The drawing under review shows one solid part. Ordinate dimensions are in mm from its lowest x, y, z. Round coordinates to 2 decimals unless told otherwise and drop trailing zeros. Order: outer loops, then holes, each group sorted by start corner. A loop starts at its lowest first (then second) coordinate and runs counter-clockwise, first axis right, second up. Notation, with made-up numbers: (66.5, 6.25) -> (89.5, 6.25) arc R25 cw to (89.5, 31.25) -> close; hole circle Ø11 at (-30.75, 67). An arc over 180 degrees is marked (long way). Use a Markdown table: item, result. Add a question column.
1) Consider section A-A (z = 2.5). State the section outline as (x, y) points, plus the area to 3 significant figures.
2) Wall thickness on line 1 along X through (y, z) = (3.3, 3.3); line 2 along Z through (x, y) = (18.5, 0.8); line 3 along Y through (x, z) = (15.5, 3.15): over which ranges is each line inside the solid? List them lowest first. Write a range as [from, to].
3) Consider section B-B (y = 3). State the section outline as (x, z) points.
4) Clearance check with a flat-ended pin moving along its axis: P1, Ø1.5, axis at x = 3.5, z = 3, coming from the +Y side. State where the tip first meets the part, or that it passes through.
5) Consider section C-C (x = 3.25). State the section outline as (y, z) points, plus the area to 3 significant figures.
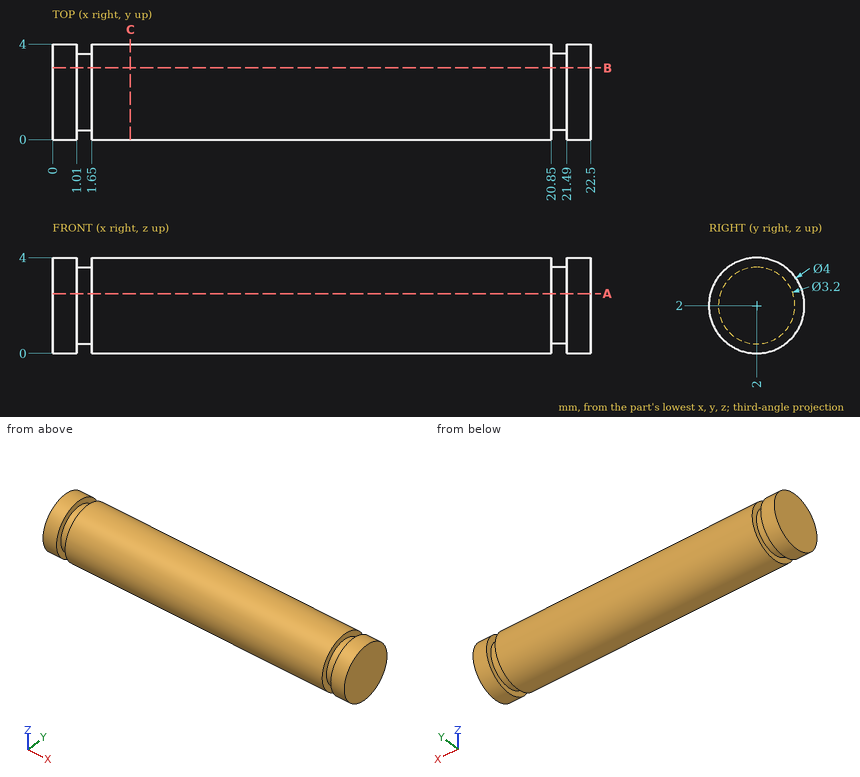
Results list:
| question | item | result |
|---|---|---|
| 1 | outline | (0, 0.06) -> (1.01, 0.06) -> (1.01, 0.48) -> (1.65, 0.48) -> (1.65, 0.06) -> (20.85, 0.06) -> (20.85, 0.48) -> (21.49, 0.48) -> (21.49, 0.06) -> (22.5, 0.06) -> (22.5, 3.94) -> (21.49, 3.94) -> (21.49, 3.52) -> (20.85, 3.52) -> (20.85, 3.94) -> (1.65, 3.94) -> (1.65, 3.52) -> (1.01, 3.52) -> (1.01, 3.94) -> (0, 3.94) -> close |
| 1 | area | 86.1 mm2 |
| 2 | line 1 | [0, 1.01], [1.65, 20.85], [21.49, 22.5] |
| 2 | line 2 | [0.4, 3.6] |
| 2 | line 3 | [0.36, 3.64] |
| 3 | outline | (0, 0.27) -> (1.01, 0.27) -> (1.01, 0.75) -> (1.65, 0.75) -> (1.65, 0.27) -> (20.85, 0.27) -> (20.85, 0.75) -> (21.49, 0.75) -> (21.49, 0.27) -> (22.5, 0.27) -> (22.5, 3.73) -> (21.49, 3.73) -> (21.49, 3.25) -> (20.85, 3.25) -> (20.85, 3.73) -> (1.65, 3.73) -> (1.65, 3.25) -> (1.01, 3.25) -> (1.01, 3.73) -> (0, 3.73) -> close |
| 4 | P1 | y = 3.98 |
| 5 | outline | circle Ø4 at (2, 2) |
| 5 | area | 12.6 mm2 |
